Model file for the job. Use its own axes, mm. A direction names the side the tool comes from. Give positions to 0.01 mm unless a question says otherwise; leave off trailing zeros. Write each loop counter-clockwise with the first axis right and the second up, starting at its lowest first coordinate (ties: lowest second). Pieces come first, ordered by that corner, then holes. Notation, with made-up numbers: (49.5, -18.5) - (88.5, -18.5) arc R13 ccw to (88.5, -2.5) - close; hole circle Ø8 at (-2, 5). An arc over 180 degrees is marked (long way). One line per item, written item: value. Start each with the question number.
(1) Cut at A-A, the plane z = -1.75. List the corners of the cut face in (x, y), and give its area (3 significant figures).
(2) 3-axis set-ups, long thin cutter, end or side, ignore diameter. For faces 1 (the face through (-31.516, 25.412, 1.326)), 2 (the face through (-23.596, 22, 1)), 3 (the face through (-46.196, 9, 1)): which of +Z, -Z, +X, -X, +Y, -Y reach the whole face in a straight line?
(3) Cut at B-B, the plane x = -41. List the corners of the cut face in (y, z).
(4) Drop flat-ended pins along their axis: P1, Ø2, axis at y = 6, z = 5, coming from the +X side; P2, Ø4, axis at x = -37, y = 23.5, coming from the +Z side; P3, Ø1, axis at x = -37, z = 3.5, coming from the +Y side; P4, Ø3.5, axis at x = -21.5, z = 4, coming from the +Y side. Give the stop position or say it passes through.
(5) Cut at C-C, the plane y = 9. List the corners of the cut face in (x, z), and give its area (3 significant figures).
(6) Mould opens along Z. For faces 4 (the face through (-35, 11, 7.257)), 5 (the face through (-23.596, 9, 1)), 6 (the face through (-50, 19, 1.677)) say: pulls with the +Z half, pulls with the -Z half, needs draft (parallel to the pull), parting line crosses it, or undercut.
(7) Probe L1, parallel to Y at x = -41.5, z = 5.75; L2, parallel to Y at x = -46, z = 3.25; L3, parallel to X at y = 10.5, z = -3.75. List the from-to ranges inside material, lowest first.
(8) Cut at D-D, the plane x = -25. List the corners of the cut face in (y, z), and give its area (3 significant figures).
from build123d import *

# Parameters (mm, degrees)
SKETCH1_W            = 22.6
SKETCH1_H            = 12
BOSS_EXTRUDE1_DEPTH  = 22.7
SKETCH4_R            = 5.84
BOSS_EXTRUDE6_DEPTH  = 5.5
SKETCH12_R           = 2.335
BOSS_EXTRUDE7_DEPTH  = 4
SKETCH13_R           = 2.5
BOSS_EXTRUDE8_DEPTH  = 5.5
SKETCH14_W           = 12
SKETCH14_H           = 2.5
BOSS_EXTRUDE10_DEPTH = 4.5
SKETCH15_R           = 1
SKETCH15_W           = 1.5
SKETCH15_H           = 0.84
CUT_EXTRUDE3_DEPTH   = 52.05819482
SKETCH16_W           = 12
SKETCH16_H           = 2.5
BOSS_EXTRUDE11_DEPTH = 4.5
SKETCH17_R           = 1
SKETCH17_W           = 1.5
SKETCH17_H           = 0.84
CUT_EXTRUDE4_DEPTH   = 56.162931847


with BuildPart() as part:
    # Sketch1 → Boss-Extrude1 (new body)
    with BuildSketch(Plane(origin=(0, 0, 0), x_dir=(1, 0, 0), z_dir=(0, 1, 0))):
        with Locations((-34.895532414, -1.256861806)):
            Rectangle(SKETCH1_W, SKETCH1_H)
    extrude(amount=BOSS_EXTRUDE1_DEPTH)

    # Sketch4 → Boss-Extrude6 (add)
    with BuildSketch(Plane(origin=(0, 22.7, 0), x_dir=(-1, 0, 0), z_dir=(0, 1, 0))):
        with Locations((40.355532414, 1.256861806)):
            Circle(SKETCH4_R)
    extrude(amount=BOSS_EXTRUDE6_DEPTH)

    # Sketch12 → Boss-Extrude7 (add)
    with BuildSketch(Plane(origin=(0, 28.2, 0), x_dir=(-1, 0, 0), z_dir=(0, 1, 0))):
        with Locations(Location((40.355532414, 1.256861806, 0), (0, 0, 90))):
            Circle(SKETCH12_R)
    extrude(amount=BOSS_EXTRUDE7_DEPTH)

    # Sketch13 → Boss-Extrude8 (add)
    with BuildSketch(Plane(origin=(0, 22.7, 0), x_dir=(-1, 0, 0), z_dir=(0, 1, 0))):
        with Locations((34.015532414, 1.256861806)):
            Circle(SKETCH13_R)
    extrude(amount=BOSS_EXTRUDE8_DEPTH)

    # Sketch14 → Boss-Extrude10 (add)
    with BuildSketch(Plane(origin=(-23.595532414, 0, 0), x_dir=(0, 0, -1), z_dir=(1, 0, 0))):
        with Locations((-1.256861806, 19.25)):
            Rectangle(SKETCH14_W, SKETCH14_H)
    extrude(amount=BOSS_EXTRUDE10_DEPTH)

    # Sketch15 → Cut-Extrude3 (cut, through all)
    with BuildSketch(Plane(origin=(0, 20.5, 0), x_dir=(-1, 0, 0), z_dir=(0, 1, 0))):
        with Locations((21.395532414, 1.256861806)):
            Circle(SKETCH15_R)
        with Locations((48.395532414, 1.256861806)):
            Circle(SKETCH15_R)
        with Locations((19.845532414, 1.256861806)):
            Rectangle(SKETCH15_W, SKETCH15_H)
    extrude(amount=-CUT_EXTRUDE3_DEPTH, mode=Mode.SUBTRACT)

    # Sketch16 → Boss-Extrude11 (add)
    with BuildSketch(Plane.ZY.offset(46.195532414)):
        with Locations((1.256861806, 19.25)):
            Rectangle(SKETCH16_W, SKETCH16_H)
    extrude(amount=BOSS_EXTRUDE11_DEPTH)

    # Sketch17 → Cut-Extrude4 (cut, through all)
    with BuildSketch(Plane(origin=(0, 20.5, 0), x_dir=(-1, 0, 0), z_dir=(0, 1, 0))):
        with Locations((48.295532414, 1.256861806)):
            Circle(SKETCH17_R)
        with Locations((49.945532414, 1.256861806)):
            Rectangle(SKETCH17_W, SKETCH17_H)
    extrude(amount=-CUT_EXTRUDE4_DEPTH, mode=Mode.SUBTRACT)


solid = part.part
Answers follow:
1. outline: (-50.7, 18) - (-46.2, 18) - (-46.2, 0) - (-23.6, 0) - (-23.6, 18) - (-19.1, 18) - (-19.1, 20.5) - (-23.6, 20.5) - (-23.6, 22.7) - (-35.35, 22.7) - (-35.35, 28.2) - (-45.36, 28.2) - (-45.36, 22.7) - (-46.2, 22.7) - (-46.2, 20.5) - (-50.7, 20.5) - close
1. area: 591 mm²
2. face 1: +Y
2. face 2: +Z, -Z, +X, +Y
2. face 3: +Z, -Z, -X, -Y
3. outline: (0, -4.74) - (22.7, -4.74) - (22.7, -4.55) - (28.2, -4.55) - (28.2, -0.99) - (32.2, -0.99) - (32.2, 3.5) - (28.2, 3.5) - (28.2, 7.06) - (22.7, 7.06) - (22.7, 7.26) - (0, 7.26) - close
4. P1: stops at x = -23.6
4. P2: stops at z = 7.26
4. P3: stops at y = 28.2
4. P4: stops at y = 20.5
5. outline: (-46.2, -4.74) - (-23.6, -4.74) - (-23.6, 7.26) - (-46.2, 7.26) - close
5. area: 271 mm²
6. face 4: pulls with the +Z half
6. face 5: needs draft
6. face 6: undercut
7. L1: y = 0 to 28.2
7. L2: y = 0 to 22.7
7. L3: x = -46.2 to -23.6
8. outline: (0, -4.74) - (22.7, -4.74) - (22.7, 7.26) - (0, 7.26) - close
8. area: 272 mm²
